Geometry: final body of the model. Coordinates: model frame, mm. A direction names the side the tool comes from. Coordinates: 2 decimals unless noted, no trailing zeros. Loops run counter-clockwise (first coordinate to the right, second up) from the corner with the lowest first, then second, coordinate; pieces in that order, holes last. Notation, with made-up numbers: (15.5, 30.5) -> (70.5, 30.5) arc R24 ccw to (70.5, 52.5) -> close; hole circle Ø8 at (13, 84). An arc over 180 degrees is marked (long way). One line per item, written item: value. Start each with the question number.
Item 1: Ray query, probe 1 along X at (y, z) = (21, 2.75); probe 2 along Z at (x, y) = (-18, 58.5); probe 3 along X at (y, z) = (59, 9). Return the intervals inside material, ascending. Write a range as from..to.
Item 2: Section query D-D on y = 55. Return loops of the section in (x, z), then the cut area to 3 significant figures.
Item 3: Contact query for flat-ended pins moving along their axis: pin 1 Ø12 at (x, y) = (-23.5, 27) entering from +Z; pin 2 Ø1.5 at (x, y) = (-11.5, 51.5) entering from -Z; pin 3 Ø4 at (x, z) = (-21.5, 3.5) entering from -Y. Output: stop coordinate, or through.
Item 4: Set-up query: faces 4 (the flat face through (-33, 17, 9)), 5 (the flat face through (-36, 37, 9)). Return all of +Z, -Z, +X, -X, +Y, -Y with unobstructed straight access to the full face (end or side cutting, diameter ignored); none if empty.
Item 5: Section query C-C on y = 30. Return loops of the section in (x, z), then the cut area to 3 significant figures.
Item 6: Section query A-A on z = 9. Return loops of the section in (x, y), then the cut area to 3 significant figures.
Item 7: Mould query, pull axis Y, two halves, no side actions, for faces 1 (the cylindrical face through (-13.181, 49.205, 14.874)), 2 (the flat face through (-3, 18, 9)), 3 (the cylindrical face through (-35.4, 73.43, 9.13)). Classes: +Y half, -Y half, draft (parallel to the pull), parting line (faces both ways), or undercut.
from build123d import *

# Parameters (mm, degrees)
BOSS_EXTRUDE1_DEPTH     = 18
CUT_EXTRUDE1_REACH      = 86.238
CUT_EXTRUDE1_END_RADIUS = 15
SKETCH3_R               = 7
FILLET1_R               = 2
FILLET2_R               = 2


with BuildPart() as part:
    # Sketch2 → Boss-Extrude1 (new body)
    with BuildSketch(Plane.XY):
        with BuildLine():
            Line((-33.38706816, 74), (-36, 74))
            Line((-36, 74), (-36, 0))
            Line((-36, 0), (-33, 0))
            Line((-33, 0), (-33, 35))
            ThreePointArc((-33, 35), (-18, 50), (-3, 35))
            Line((-3, 35), (-3, 0))
            Line((-3, 0), (0, 0))
            Line((0, 0), (0, 74))
            Line((0, 74), (-12.61679677, 74))
            Line((-12.61679677, 74), (-33.38706816, 74))
        make_face()
    extrude(amount=BOSS_EXTRUDE1_DEPTH)

    # Cut-Extrude1: up to this cylinder (the profile starts outside it)
    cut_extrude1_end = Plane(origin=(-18, 35, 9), z_dir=(0, 0, -1)) * Cylinder(CUT_EXTRUDE1_END_RADIUS, 203.476, mode=Mode.PRIVATE)
    # Sketch3 → Cut-Extrude1 (cut, up to the surface)
    with BuildSketch(Plane(origin=(0, 74, 0), x_dir=(1, 0, 0), z_dir=(0, 1, 0)), mode=Mode.PRIVATE) as cut_extrude1_sk1:
        with Locations(Location((-18, -9, 0), (0, 0, 270))):
            Circle(SKETCH3_R)
    cut_extrude1_tool1 = extrude(cut_extrude1_sk1.sketch, amount=-CUT_EXTRUDE1_REACH, mode=Mode.PRIVATE) - cut_extrude1_end
    add(cut_extrude1_tool1.solids().sort_by_distance((-18, 74, 9))[0], mode=Mode.SUBTRACT)

    # Fillet1
    fillet1_edges = [part.edges().sort_by_distance(p)[0] for p in [
        (-18, 74, 2),
    ]]
    fillet(fillet1_edges, radius=FILLET1_R - 0.0001)  # a hair under: the kernel refuses the full size

    # Fillet2
    fillet2_edges = [part.edges().sort_by_distance(p)[0] for p in [
        (-36, 74, 9),
        (0, 74, 9),
    ]]
    fillet(fillet2_edges, radius=FILLET2_R)


solid = part.part
Reply:
1. probe 1: x = -36..-33, -3..0
1. probe 2: z = 0..2, 16..18
1. probe 3: x = -36..-25, -11..0
2. outline: (-36, 0) -> (0, 0) -> (0, 18) -> (-36, 18) -> close; hole circle Ø14 at (-18, 9)
2. area: 494 mm²
3. pin 1: passes through
3. pin 2: stops at z = 0
3. pin 3: stops at y = 48.96
4. face 4: +Z, -Z, -Y
4. face 5: +Z, -Z, -X, +Y, -Y
5. outline: (-36, 0) -> (-33, 0) -> (-33, 18) -> (-36, 18) -> close; (-3, 0) -> (0, 0) -> (0, 18) -> (-3, 18) -> close
5. area: 108 mm²
6. outline: (-36, 0) -> (-33, 0) -> (-33, 35) arc R15 cw to (-25, 48.27) -> (-25, 72) arc R2 ccw to (-27, 74) -> (-34, 74) arc R2 ccw to (-36, 72) -> close; (-11, 48.27) arc R15 cw to (-3, 35) -> (-3, 0) -> (0, 0) -> (0, 72) arc R2 ccw to (-2, 74) -> (-9, 74) arc R2 ccw to (-11, 72) -> close
6. area: 913 mm²
7. face 1: -Y half
7. face 2: draft
7. face 3: +Y half
